from build123d import *

# Parameters (mm, degrees)
EXTRUDE_THIN1_DEPTH = 4.8
SKETCH2_R           = 2.1
CUT_EXTRUDE1_DEPTH  = 41.792156109
SKETCH3_R           = 2.1
CUT_EXTRUDE2_DEPTH  = 42.07359249
FILLET1_R           = 4.8


with BuildPart() as part:
    # Sketch1 → Extrude-Thin1 (new body)
    with BuildSketch(Plane.XY):
        with BuildLine():
            Line((0, -0.8), (11.691868154, -0.8))
            ThreePointArc((11.691868154, -0.8), (12.145726205, -0.756695328), (12.583205778, -0.628344058))
            Line((12.583205778, -0.628344058), (28.011019305, 5.542781353))
            ThreePointArc((28.011019305, 5.542781353), (28.156845829, 5.585565109), (28.308131846, 5.6))
            Line((28.308131846, 5.6), (40, 5.6))
            Line((40, 5.6), (40, 7.2))
            Line((40, 7.2), (28.308131846, 7.2))
            ThreePointArc((28.308131846, 7.2), (27.854273795, 7.156695328), (27.416794222, 7.028344058))
            Line((27.416794222, 7.028344058), (11.988980695, 0.857218647))
            ThreePointArc((11.988980695, 0.857218647), (11.843154171, 0.814434891), (11.691868154, 0.8))
            Line((11.691868154, 0.8), (0, 0.8))
            Line((0, 0.8), (0, -0.8))
        make_face()
    extrude(amount=EXTRUDE_THIN1_DEPTH)

    # Sketch2 → Cut-Extrude1 (cut, through all)
    with BuildSketch(Plane(origin=(0, 0.8, 0), x_dir=(1, 0, 0), z_dir=(0, 1, 0))):
        with Locations((4, 0)):
            Circle(SKETCH2_R)
    extrude(amount=-CUT_EXTRUDE1_DEPTH, mode=Mode.SUBTRACT)

    # Sketch3 → Cut-Extrude2 (cut, through all)
    with BuildSketch(Plane(origin=(0, 7.2, 0), x_dir=(1, 0, 0), z_dir=(0, 1, 0))):
        with Locations((36, 0)):
            Circle(SKETCH3_R)
    extrude(amount=-CUT_EXTRUDE2_DEPTH, mode=Mode.SUBTRACT)

    # Fillet1
    fillet1_edges = [part.edges().sort_by_distance(p)[0] for p in [
        (0, 0, 4.8),
        (40, 6.4, 4.8),
    ]]
    fillet(fillet1_edges, radius=FILLET1_R - 0.0001)  # a hair under: the kernel refuses the full size

    # Mirror1: part across plane


with BuildPart() as part_1:
    add(part.part)
    add(part.part.mirror(Plane(origin=(28.308131846, 4.8, 0), x_dir=(1, 0, 0), z_dir=(0, 0, 1))))


solid = part_1.part
The model under review builds one solid part; all positions refer to its coordinate system, in mm. A direction names the side the tool comes from. Give positions to 0.01 mm unless a question says otherwise; leave off trailing zeros. Write each loop counter-clockwise with the first axis right and the second up, starting at its lowest first coordinate (ties: lowest second). Pieces come first, ordered by that corner, then holes.
1. For P1, Ø2, axis at x = 28.5, y = 4, coming from the -Z side; P2, Ø3, axis at x = 25.5, z = 0, coming from the -Y side; P3, Ø5, axis at x = 5, z = 1, coming from the +Y side, all flat-tipped, find the tip position at first contact; note any pin that passes through.
2. Add section B-B, the plane x = 4. Write out the cut boundary in (y, z), plus the area to 3 significant figures.
3. Wall thickness on L1, parallel to Y at x = 10, z = 2.5; L2, parallel to Z at x = 36, y = 6.8; L3, parallel to X at y = 6, z = 1.5: over which ranges is each line inside the solid? List them lowest first.
4. Add section D-D, the plane x = 9.5. Write out the cut boundary in (y, z), plus the area to 3 significant figures.
5. Add section C-C, the plane z = 3. Write out the cut boundary in (x, y).
6. Add section A-A, the plane z = -1.5. Write out the cut boundary in (x, y).
7. Draft analysis for pull direction X (two halves, no side actions). For faces 3 (the flat face through (33, 5.6, 0)), 4 (the cylindrical face through (33.9, 6.41, 0.09)), 5 (the cylindrical face through (1.44, -0.01, -3.43)), state which applies: +X half, -X half, draft (parallel to the pull), parting line (faces both ways), or undercut.
8. Tool access review of faces 1 (the cylindrical face through (38.56, 6.41, 3.43)), 2 (the flat face through (7, 0.8, 0)): name each direction out of +Z, -Z, +X, -X, +Y, -Y from which nothing blocks a thin tool from reaching the whole face with its end or side.
Worked answers:
1. P1: passes through
1. P2: stops at y = 3.94
1. P3: stops at y = 0.8
2. outline: (-0.8, -4.73) - (0.8, -4.73) - (0.8, -2.1) - (-0.8, -2.1) - close; (-0.8, 2.1) - (0.8, 2.1) - (0.8, 4.73) - (-0.8, 4.73) - close
2. area: 8.43 mm2
3. L1: y = -0.8 to 0.8
3. L2: z = -4.73 to -2.1, 2.1 to 4.73
3. L3: x = 24.85 to 34.53, 37.47 to 39.76
4. outline: (-0.8, -4.8) - (0.8, -4.8) - (0.8, 4.8) - (-0.8, 4.8) - close
4. area: 15.4 mm2
5. outline: (1.05, -0.8) - (11.69, -0.8) arc R2.4 ccw to (12.58, -0.63) - (28.01, 5.54) arc R0.8 cw to (28.31, 5.6) - (38.95, 5.6) - (38.95, 7.2) - (28.31, 7.2) arc R2.4 ccw to (27.42, 7.03) - (11.99, 0.86) arc R0.8 cw to (11.69, 0.8) - (1.05, 0.8) - close
6. outline: (0.24, -0.8) - (2.53, -0.8) - (2.53, 0.8) - (0.24, 0.8) - close; (5.47, -0.8) - (11.69, -0.8) arc R2.4 ccw to (12.58, -0.63) - (28.01, 5.54) arc R0.8 cw to (28.31, 5.6) - (34.53, 5.6) - (34.53, 7.2) - (28.31, 7.2) arc R2.4 ccw to (27.42, 7.03) - (11.99, 0.86) arc R0.8 cw to (11.69, 0.8) - (5.47, 0.8) - close; (37.47, 5.6) - (39.76, 5.6) - (39.76, 7.2) - (37.47, 7.2) - close
7. face 3: draft
7. face 4: undercut
7. face 5: -X half
8. face 1: +Z, +X, +Y, -Y
8. face 2: +Z, -Z, -X, +Y
